Work out the finished part from the listing and answer in its coordinate system (mm). A direction names the side the tool comes from. Give positions to 0.01 mm unless a question says otherwise; leave off trailing zeros. Loops run counter-clockwise (first coordinate to the right, second up) from the corner with the lowest first, then second, coordinate; pieces in that order, holes last. Notation, with made-up numbers: M 37.25,53 L 74.25,53 A31 cw 74.25,81 Z; hole C -16.5,89.5 d7. An arc over 180 degrees is marked long. Use a Markdown table: item, result.
Autodesk Inventor part; units mm, degrees
ref_plane "YZ Plane" through (0, 0, 0) normal (1, 0, 0) x (0, 1, 0)
ref_plane "XZ Plane" through (0, 0, 0) normal (0, 1, 0) x (-1, 0, 0)
ref_plane "XY Plane" through (0, 0, 0) normal (0, 0, 1) x (1, 0, 0)
sketch "スケッチ1" plane through (0, 0, 0) normal (1, 0, 0) x (0, 1, 0)
  line L0 (0, 0) -> (21.05, 0)
  line L1 (21.05, 0) -> (21.05, -53.5)
  line L2 (21.05, -53.5) -> (0, -53.5)
  line L3 (0, -53.5) -> (0, 0)
  line L4 (0, -53.5) -> (7.5, -53.5)
  line L5 (7.5, -53.5) -> (7.5, -57.8)
  line L6 (7.5, -57.8) -> (0, -57.8)
  line L7 (0, -57.8) -> (0, -53.5)
  line L8 (0, -57.8) -> (2.5, -57.8)
  line L9 (2.5, -57.8) -> (2.5, -71.1)
  line L10 (2.5, -71.1) -> (0, -71.1)
  line L11 (0, -71.1) -> (0, -57.8)
  line L12 (0, 0) -> (7.5, 0)
  line L13 (7.5, 0) -> (7.5, 4.4)
  line L14 (7.5, 4.4) -> (0, 4.4)
  line L15 (0, 4.4) -> (0, 0)
  line L16 (0, 4.4) -> (2.5, 4.4)
  line L17 (2.5, 4.4) -> (2.5, 11.9)
  line L18 (2.5, 11.9) -> (0, 11.9)
  line L19 (0, 11.9) -> (0, 4.4)
  line L20 (0, -4.9) -> (22.5, -4.9)
  line L21 (22.5, -4.9) -> (22.5, -31.9)
  line L22 (22.5, -31.9) -> (0, -31.9)
  line L23 (0, -31.9) -> (0, -4.9)
  point P0 (1.25, -71.1)
  point P1 (3.75, -53.5)
  point P2 (21.05, -4.9)
  point P3 (21.05, -31.9)
  dimension "d0" = 2.5
  dimension "d1" = 11.9
  dimension "d2" = 4.4
  dimension "d3" = 7.5
  dimension "d4" = 21.05
  dimension "d5" = 22.5
  dimension "d6" = 53.5
  dimension "d8" = 17.6
  dimension "d9" = 4.3
  dimension "d10" = 2.5
  dimension "d11" = 4.9
  dimension "d12" = 27
revolve "回転1" add sketch "スケッチ1" angle 360 about axis through (0, 0, -31.9) along (0, 0, 1)
sketch "スケッチ2" plane through (0, 0, 0) normal (0, 0, 1) x (1, 0, 0)
  circle A0 centre (0, 0) radius 14.5
  point P0 (14.5, 0)
  point P1 (-14.5, 0)
  dimension "d14" = 29
hole "穴1" at (14.5, 0, 0) at (-14.5, 0, 0) direction (0, 0, -1) diameter 4 depth 8 tip angle 118
thread "ねじ1"
thread "ねじ2"
properties part number "RZ735" material "ステンレス鋼"
(1) Given P1, Ø8, axis at x = 1, y = 17, coming from the -Z side; P2, Ø6, axis at y = -16.5, z = -25.5, coming from the -X side; P3, Ø2, axis at y = 8.5, z = -17, coming from the -X side, each flat-ended and moving along its own axis, determine where each tip first touches the part or whether it passes through.
Entries:
| item | result |
|---|---|
| P1 | stops at z = -53.5 |
| P2 | stops at x = -18 |
| P3 | stops at x = -21.21 |
(2) Consider probe 1 along X at (y, z) = (0, -6); probe 2 along Z at (x, y) = (-7, -17); probe 3 along Z at (x, y) = (2, 5.5). Determine where each line is inside the solid, lowest interval first. Write a range as [from, to].
Entries:
| item | result |
|---|---|
| probe 1 | x = [-22.5, -16.5], [-12.5, 12.5], [16.5, 22.5] |
| probe 2 | z = [-53.5, 0] |
| probe 3 | z = [-57.8, 4.4] |
(3) Which of the six approach directions +Z, -Z, +X, -X, +Y, -Y give full straight-line access (tool end or side, diameter ignored) to faces 1 (the cylindrical face through (6.32, 20.08, -42.85)), 2 (the flat face through (0, 0, -71.1)), 3 (the cylindrical face through (6.32, 20.08, -2.48))?
Entries:
| item | result |
|---|---|
| face 1 | -Z |
| face 2 | -Z, +X, -X, +Y, -Y |
| face 3 | +Z |
(4) A cutting plane is placed at C-C (z = -20). Write down the section's boundary in (x, y), and give its area (3 significant figures).
Entries:
| item | result |
|---|---|
| outline | C 0,0 d45 |
| area | 1,590 mm² |
(5) A cutting plane is placed at D-D (x = -5.5). Write down the section's boundary in (y, z).
Entries:
| item | result |
|---|---|
| outline | M -21.82,-31.9 L -20.32,-31.9 L -20.32,-53.5 L -5.1,-53.5 L -5.1,-57.8 L 5.1,-57.8 L 5.1,-53.5 L 20.32,-53.5 L 20.32,-31.9 L 21.82,-31.9 L 21.82,-4.9 L 20.32,-4.9 L 20.32,0 L 5.1,0 L 5.1,4.4 L -5.1,4.4 L -5.1,0 L -20.32,0 L -20.32,-4.9 L -21.82,-4.9 Z |
(6) The mould has two halves that part along Y. Classify faces 4 (the flat face through (-2, -2, 4.4)), 5 (the cylindrical face through (-16.483, 0.26, -4.056)), 6 (the cylindrical face through (-19.961, 10.382, -18.589)): released by +Y, released by -Y, zero draft, split by the parting line, or undercut.
Entries:
| item | result |
|---|---|
| face 4 | zero draft |
| face 5 | undercut |
| face 6 | split by the parting line |
(7) A cutting plane is placed at B-B (y = 6). Write down the section's boundary in (x, z).
Entries:
| item | result |
|---|---|
| outline | M -21.69,-31.9 L -20.18,-31.9 L -20.18,-53.5 L -4.5,-53.5 L -4.5,-57.8 L 4.5,-57.8 L 4.5,-53.5 L 20.18,-53.5 L 20.18,-31.9 L 21.69,-31.9 L 21.69,-4.9 L 20.18,-4.9 L 20.18,0 L 4.5,0 L 4.5,4.4 L -4.5,4.4 L -4.5,0 L -20.18,0 L -20.18,-4.9 L -21.69,-4.9 Z |
(8) A cutting plane is placed at A-A (x = 0). Write down the section's boundary in (y, z).
Entries:
| item | result |
|---|---|
| outline | M -22.5,-31.9 L -21.05,-31.9 L -21.05,-53.5 L -7.5,-53.5 L -7.5,-57.8 L -2.5,-57.8 L -2.5,-71.1 L 2.5,-71.1 L 2.5,-57.8 L 7.5,-57.8 L 7.5,-53.5 L 21.05,-53.5 L 21.05,-31.9 L 22.5,-31.9 L 22.5,-4.9 L 21.05,-4.9 L 21.05,0 L 7.5,0 L 7.5,4.4 L 2.5,4.4 L 2.5,11.9 L -2.5,11.9 L -2.5,4.4 L -7.5,4.4 L -7.5,0 L -21.05,0 L -21.05,-4.9 L -22.5,-4.9 Z |
